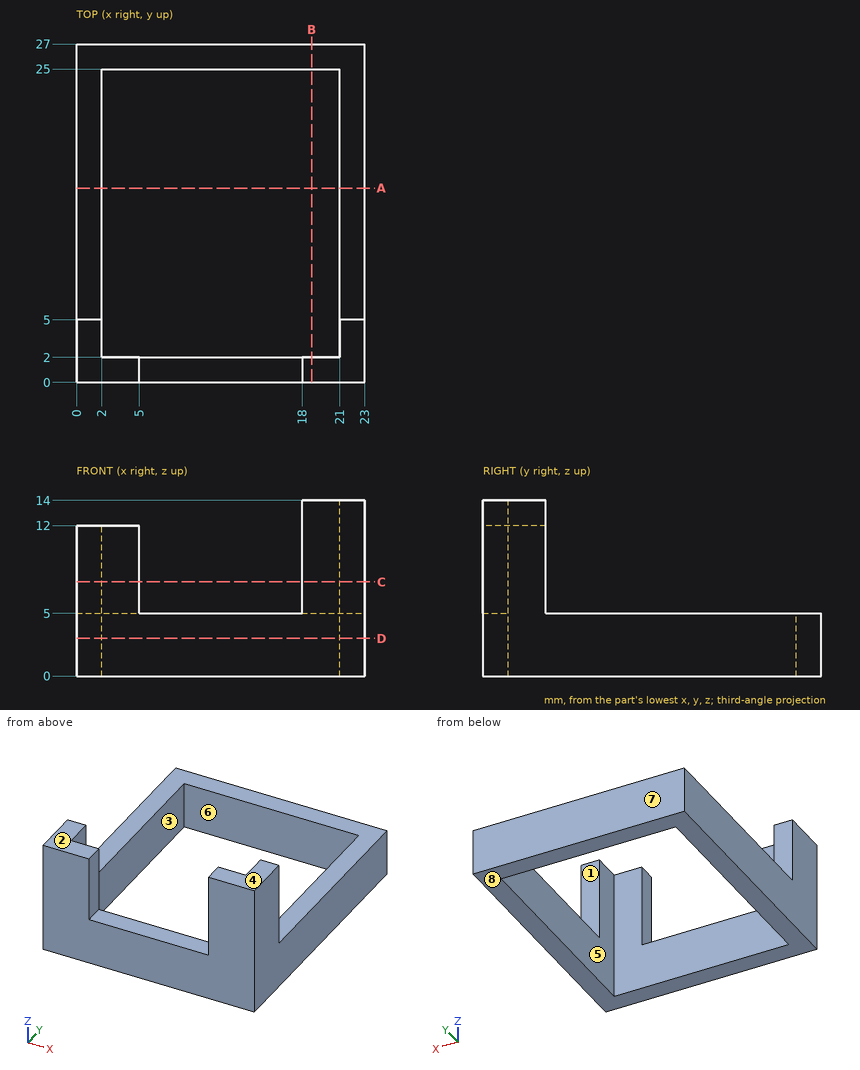
Geometry: see drawing. Coordinates: mm, zero at the bounding-box minimum. A direction names the side the tool comes from. Round coordinates to 2 decimals unless told otherwise and drop trailing zeros. Write each loop counter-clockwise with the first axis right and the second up, starting at its lowest first coordinate (ties: lowest second). Pieces come first, ordered by that corner, then holes.
1) Reachability of the marked faces 1, 2, 3 and 4 from +Z, -Z, +X, -X, +Y, -Y: full face, straight path, thin tool, end or side. Return the list, or none.
2) Cut plane A-A (y = 15.5). Return the cut outline in (x, z).
3) Cut plane C-C (z = 7.5). Return the cut outline in (x, y).
4) Draft query along Y for the marked faces 5, 6, 7 and 8. Return one class per face: pulls with the +Y half, pulls with the -Y half, needs draft (parallel to the pull), parting line crosses it, or undercut.
5) Ray query, L1, parallel to X at y = 10.25, z = 3.5; L2, parallel to Y at x = 11.75, z = 3.75; L3, parallel to Y at x = 2.25, z = 7.5. Return the intervals inside material, ascending.
6) Cut plane D-D (z = 3). Return the cut outline in (x, y), then the cut area to 3 significant figures.
7) Cut plane B-B (x = 18.75). Return the cut outline in (y, z), then the cut area to 3 significant figures.
8) Contact query for flat-ended pins moving along their axis: P1, Ø0.6, axis at x = 9, y = 0.5, coming from the +Z side; P2, Ø0.6, axis at x = 22, z = 10, coming from the +Y side; P3, Ø2.5, axis at x = 2, y = 1.5, coming from the +Z side. Output: stop coordinate, or through.
Geometry says:
1. face 1: +Z, +X, -X, +Y
1. face 2: +Z, -X, +Y, -Y
1. face 3: +Z, -Z
1. face 4: +Z, +X, -X, +Y, -Y
2. outline: (0, 0) - (2, 0) - (2, 5) - (0, 5) - close; (21, 0) - (23, 0) - (23, 5) - (21, 5) - close
3. outline: (0, 0) - (5, 0) - (5, 2) - (2, 2) - (2, 5) - (0, 5) - close; (18, 0) - (23, 0) - (23, 5) - (21, 5) - (21, 2) - (18, 2) - close
4. face 5: undercut
4. face 6: undercut
4. face 7: pulls with the +Y half
4. face 8: needs draft
5. L1: x = 0 to 2, 21 to 23
5. L2: y = 0 to 2, 25 to 27
5. L3: y = 0 to 2
6. outline: (0, 0) - (23, 0) - (23, 27) - (0, 27) - close; hole (2, 2) - (21, 2) - (21, 25) - (2, 25) - close
6. area: 184 mm2
7. outline: (0, 0) - (2, 0) - (2, 14) - (0, 14) - close; (25, 0) - (27, 0) - (27, 5) - (25, 5) - close
7. area: 38.0 mm2
8. P1: stops at z = 5
8. P2: stops at y = 5
8. P3: stops at z = 12
